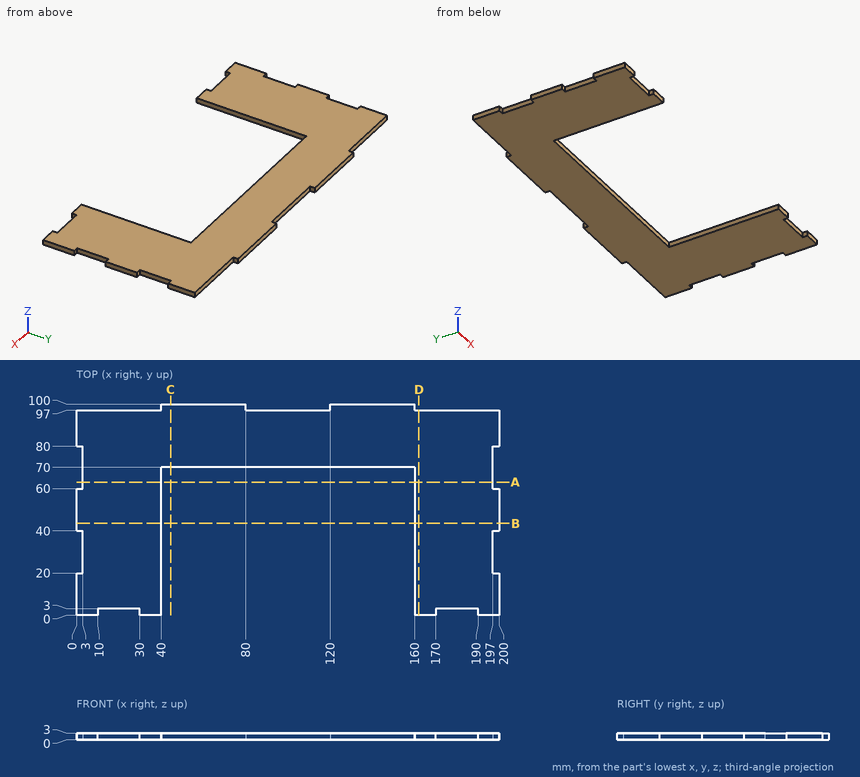
Drawing for the job (mm, zero at the part's lowest x, y, z). Coordinates: 2 decimals unless noted, no trailing zeros. Order: outer loops, then holes, each group sorted by start corner. A loop starts at its lowest first (then second) coordinate and runs counter-clockwise, first axis right, second up. Notation, with made-up numbers: (-21.5, -6.5) - (6.5, -6.5) arc R26 cw to (6.5, 19.5) - close; hole circle Ø4 at (-33.5, 17). An arc over 180 degrees is marked (long way). Use a Markdown table: item, result. Add a question column.
(1) Flat gauge pins, fed straight in: pin 1 (1.5 mm diameter, centred on y = 99, z = 1.5, fed in from +X); pin 2 (1 mm diameter, centred on y = 76, z = 1, fed in from -X); pin 3 (0.9 mm diameter, centred on x = 182, z = 2, fed in from -Y); pin 4 (10 mm diameter, centred on x = 158, y = 34, fed in from -Z). Where does each tip first touch, or does it go through?
(2) Drill centre lines: line 1 along X through (y, z) = (21.5, 0.6); line 2 along X through (y, z) = (6, 1.65); line 3 along Y through (x, z) = (92, 1.05). Where is each one in solid material? Low to high. Write a range as [from, to].
(3) Saw through at A-A (y = 63). Give the cut face in (x, z).
(4) Saw through at D-D (x = 162). Give the cut face in (y, z).
(5) Saw through at C-C (x = 44.5). Give the cut face in (y, z), then the cut area to 3 significant figures.
(6) Saw through at B-B (y = 43.5). Give the cut face in (x, z).
Solved:
| question | item | result |
|---|---|---|
| 1 | pin 1 | stops at x = 160 |
| 1 | pin 2 | stops at x = 3 |
| 1 | pin 3 | stops at y = 3 |
| 1 | pin 4 | stops at z = 0 |
| 2 | line 1 | x = [3, 40], [160, 197] |
| 2 | line 2 | x = [0, 40], [160, 200] |
| 2 | line 3 | y = [70, 97] |
| 3 | outline | (3, 0) - (40, 0) - (40, 3) - (3, 3) - close; (160, 0) - (197, 0) - (197, 3) - (160, 3) - close |
| 4 | outline | (0, 0) - (97, 0) - (97, 3) - (0, 3) - close |
| 5 | outline | (70, 0) - (100, 0) - (100, 3) - (70, 3) - close |
| 5 | area | 90.0 mm² |
| 6 | outline | (0, 0) - (40, 0) - (40, 3) - (0, 3) - close; (160, 0) - (200, 0) - (200, 3) - (160, 3) - close |
